Autodesk Inventor part; units mm, degrees
ref_plane "YZ Plane" through (0, 0, 0) normal (1, 0, 0) x (0, 1, 0)
ref_plane "XZ Plane" through (0, 0, 0) normal (0, 1, 0) x (-1, 0, 0)
ref_plane "XY Plane" through (0, 0, 0) normal (0, 0, 1) x (1, 0, 0)
sketch "Sketch1" plane through (0, 0, 0) normal (0, 1, 0) x (-1, 0, 0)
  circle A0 centre (0, 0) radius 25
  line L0 (8, 21) -> (8, -21)
  line L1 (8, -21) -> (-12, -21)
  line L2 (-12, -21) -> (-12, 21)
  line L3 (-12, 21) -> (8, 21)
  line L4 (8, 10) -> (20, 10)
  line L5 (20, 10) -> (20, -10)
  line L6 (20, -10) -> (8, -10)
  dimension "d0" = 50
  dimension "d1" = 20
  dimension "d2" = 20
  dimension "d3" = 42
  dimension "d4" = 21
  dimension "d5" = 10
  dimension "d6" = 8
  dimension "d7" = 20
extrude "Extrusion1" add sketch "Sketch1" along normal blind 2 contours A0 | L0 L1 L2 L3 | L4 L5 L6 L0
extrude "Extrusion2" add sketch "Sketch1" against normal blind 5
properties part number "Battery"
Input: part model. Units: mm. Frame: model coordinates. A direction names the side the tool comes from. Coordinates: 2 decimals unless noted, no trailing zeros. Loops run counter-clockwise (first coordinate to the right, second up) from the corner with the lowest first, then second, coordinate; pieces in that order, holes last.
(1) Section A-A on x = 1. Return the cut outline in (y, z).
(2) Section B-B on y = -1. Return the cut outline in (x, z), then the cut area to 3 significant figures.
(3) First-contact query: pin 1 Ø8 at (x, z) = (-2.5, 7) entering from -Y; pin 2 Ø3 at (x, y) = (-15.5, -1) entering from +Z; pin 3 Ø1.5 at (x, y) = (-1, -2) entering from +Z; pin 4 Ø4 at (y, z) = (-1.5, -2) entering from +X. Flat tips, straight axial feed; report the tip coordinate or a pass-through.
(4) Pull-direction query (Z, two-part tool) for faces 3 (the face through (-8, -2, 16)), 4 (the face through (0, 2, 0)), 5 (the face through (-23.846, -1.451, 7.509)); classes: released by +Z, released by -Z, zero draft, split by the parting line, or undercut.
(5) Section C-C on z = 0. Return the cut outline in (x, y), then the cut area to 3 significant figures.
(6) Set-up query: faces 1 (the face through (-11, -5, -11)), 2 (the face through (2, -2, -21)). Return all of +Z, -Z, +X, -X, +Y, -Y with unobstructed straight access to the full face (end or side cutting, diameter ignored); none if empty.
(7) Material intervals for probe 1 along Y at (x, z) = (-11.5, 3); probe 2 along X at (y, z) = (-4.5, -8.5); probe 3 along Z at (x, y) = (-13.5, -2.5), sorted ascending.
Data:
1. outline: (-5, -24.98) - (2, -24.98) - (2, 24.98) - (-5, 24.98) - (-5, 21) - (0, 21) - (0, -21) - (-5, -21) - close
2. outline: circle Ø50 at (0, 0); hole (-20, -10) - (-8, -10) - (-8, -21) - (12, -21) - (12, 21) - (-8, 21) - (-8, 10) - (-20, 10) - close
2. area: 883 mm2
3. pin 1: stops at y = 0
3. pin 2: stops at z = 20.71
3. pin 3: stops at z = 25
3. pin 4: stops at x = 25
4. face 3: undercut
4. face 4: zero draft
4. face 5: split by the parting line
5. outline: (-25, -5) - (-20, -5) - (-20, 0) - (12, 0) - (12, -5) - (25, -5) - (25, 2) - (-25, 2) - close
5. area: 190 mm2
6. face 1: +Z, -Z, +X, -X, -Y
6. face 2: -Y
7. probe 1: y = 0 to 2
7. probe 2: x = -23.51 to -20, 12 to 23.51
7. probe 3: z = -21.04 to -10, 10 to 21.04
